Check sheet for the drawn part. Datum: minimum x, y, z corner. Units: mm. A direction names the side the tool comes from. Coordinates: 2 decimals unless noted, no trailing zeros. Order: outer loops, then holes, each group sorted by start corner. A loop starts at its lowest first (then second) coordinate and runs counter-clockwise, first axis right, second up. Notation, with made-up numbers: M 3,43.5 L 21,43.5 A5 cw 21,48.5 Z; hole C 83,49.5 d5. An arc over 180 degrees is marked long. Answer in a Markdown table with one row per item. Add a question column.
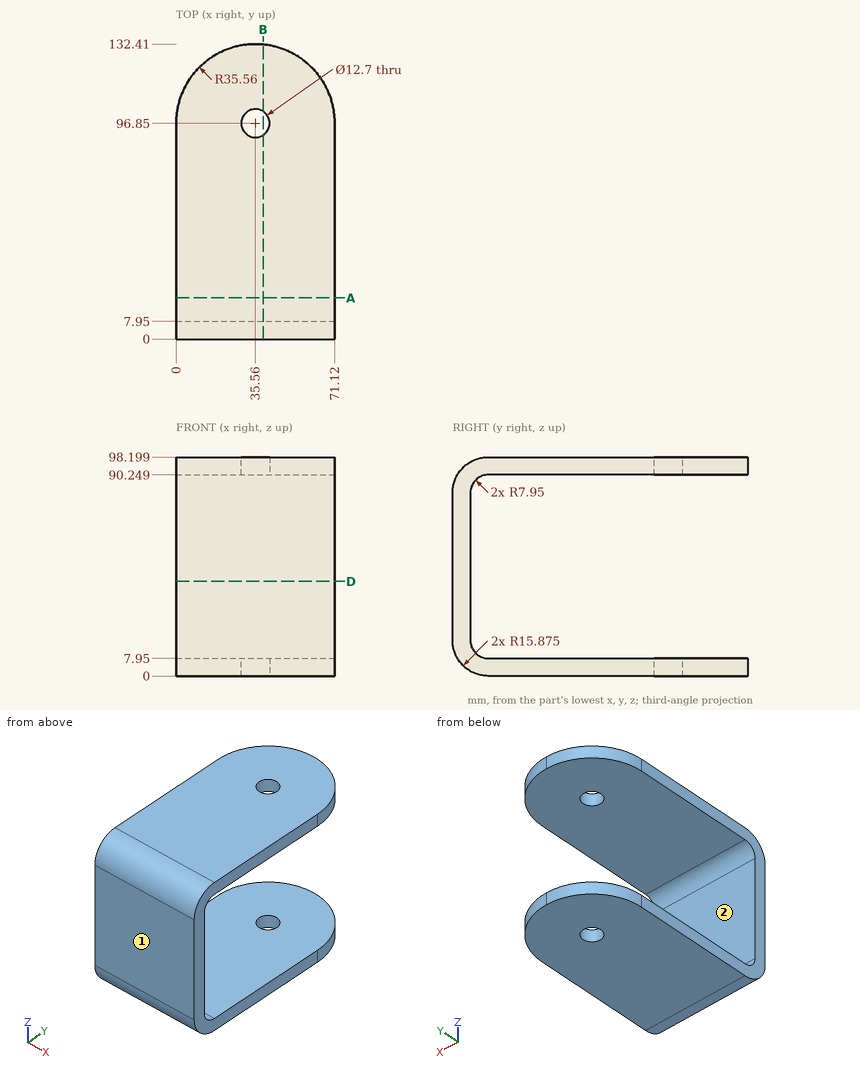
1. Section check D-D on z = 42.5. Enter the section's corners in (x, y).
2. Go/stop test with flat-tipped pins: pin 1 Ø1.5 at (x, z) = (47.5, 64) entering from +Y; pin 2 Ø12 at (x, z) = (15, 80) entering from +Y (1 decimal). Record where each tip stops, or that it passes through.
3. Section check B-B on x = 39. State how many separate pieces and enclosed holes the cut face has, then the cut area to 3 significant figures.
4. Section check A-A on y = 18.5. Enter the section's corners in (x, z).
5. Set-up check for the marked faces 1 and 2: record each of +Z, -Z, +X, -X, +Y, -Y from which the full face is reachable in a straight line by a thin tool's end or side.
6. Scan lines: line 1 (Z direction, x = 63, y = 108); line 2 (Y direction, x = 19, z = 17); line 3 (Y direction, x = 35.56, z = 4). Record each from-to range of solid material in increasing order.
Result sheet:
| question | item | result |
|---|---|---|
| 1 | outline | M 0,0 L 71.12,0 L 71.12,7.95 L 0,7.95 Z |
| 2 | pin 1 | y = 7.95 |
| 2 | pin 2 | y = 8.9 |
| 3 | separate pieces | 3 |
| 3 | enclosed holes | 0 |
| 3 | area | 2,510 mm^2 |
| 4 | outline | M 0,0 L 71.12,0 L 71.12,7.95 L 0,7.95 Z; M 0,90.25 L 71.12,90.25 L 71.12,98.2 L 0,98.2 Z |
| 5 | face 1 | +Z, -Z, +X, -X, -Y |
| 5 | face 2 | +X, -X, +Y |
| 6 | line 1 | 0 to 7.95, 90.25 to 98.2 |
| 6 | line 2 | 0 to 7.95 |
| 6 | line 3 | 5.34 to 90.5, 103.2 to 132.41 |
